For this review, use the dimensioned drawing (mm, ordinates from the lowest corner) and the shaded views. Coordinates: 2 decimals unless noted, no trailing zeros. Loops run counter-clockwise (first coordinate to the right, second up) from the corner with the lowest first, then second, coordinate; pieces in that order, holes last. Notation, with made-up numbers: (-30, -26) -> (-20, -26) arc R23 cw to (-20, 11) -> close; hole circle Ø3 at (48.25, 66.5). An arc over 180 degrees is marked (long way). Use one line per item in the form item = value. Start each with the question number.
1. Consider section B-B (y = 100). State the section outline as (x, z) points.
2. Wall thickness on line 1 (Y direction, x = 100, z = 1.75); line 2 (Y direction, x = 108, z = 2) (1 decimal); line 3 (X direction, y = 102, z = 1.05) (1 decimal): over which ranges is each line inside the solid? List them lowest first. Write a range as from..to.
3. Consider section A-A (x = 20). State the section outline as (y, z) points.
4. For pin 1 (12 mm diameter, centred on x = 160.5, y = 39, fed in from +Z); pin 2 (16 mm diameter, centred on x = 100, y = 20, fed in from +Z); pin 3 (1.5 mm diameter, centred on x = 27.5, z = 2.5, fed in from +Y) (1 decimal), all flat-tipped, find the tip position at first contact; note any pin that passes through.
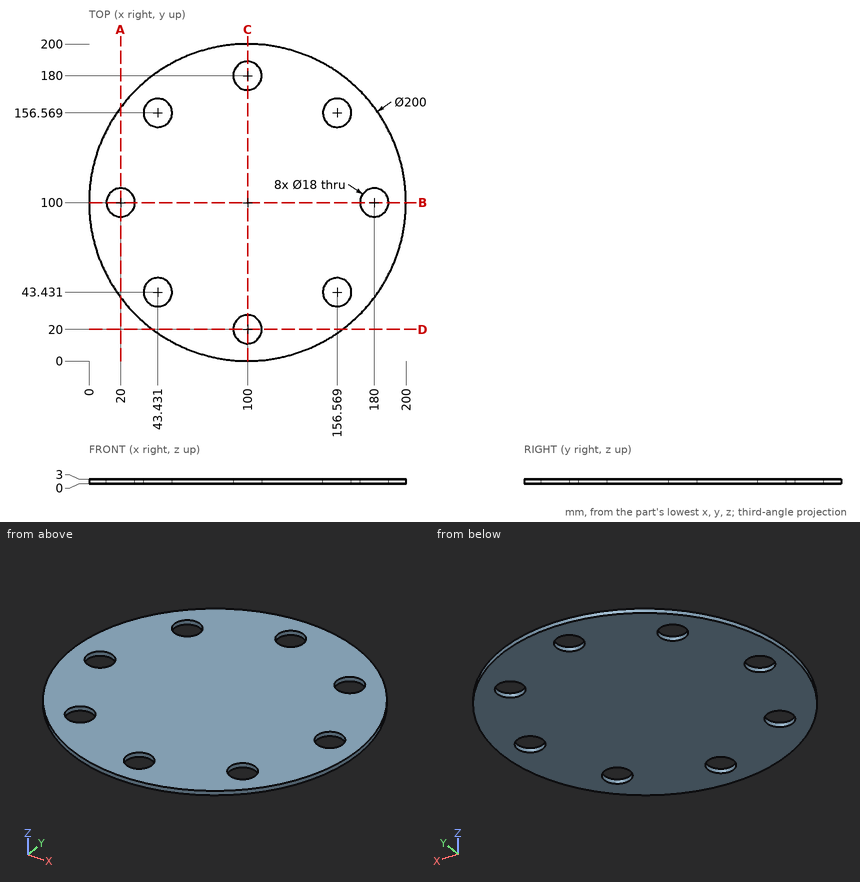
Geometry check:
q1.outline = (0, 0) -> (11, 0) -> (11, 3) -> (0, 3) -> close; (29, 0) -> (171, 0) -> (171, 3) -> (29, 3) -> close; (189, 0) -> (200, 0) -> (200, 3) -> (189, 3) -> close
q2.line_1 = 0..11, 29..171, 189..200
q2.line_2 = 0.3..15.9, 24.1..175.9, 184.1..199.7
q2.line_3 = 0..11.2, 28.8..171.2, 188.8..200
q3.outline = (40, 0) -> (91, 0) -> (91, 3) -> (40, 3) -> close; (109, 0) -> (160, 0) -> (160, 3) -> (109, 3) -> close
q4.pin_1 = 3
q4.pin_2 = through
q4.pin_3 = 169.7
